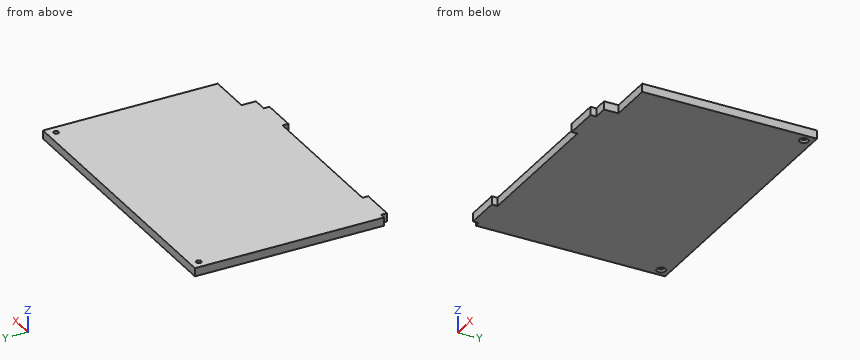
from build123d import *

# Parameters (mm, degrees)
BOSS_EXTRUDE1_DEPTH                             = 5.9
MOVE_FACE1_BY                                   = 6.3
CSK_FOR_M3_FLAT_HEAD_MACHINE_SCREW2_D           = 3.6
CSK_FOR_M3_FLAT_HEAD_MACHINE_SCREW2_CSINK_D     = 6.3
CSK_FOR_M3_FLAT_HEAD_MACHINE_SCREW2_CSINK_ANGLE = 90


with BuildPart() as part:
    # Sketch1 → Boss-Extrude1 (new body)
    with BuildSketch(Plane.XY):
        Polygon((0, 0), (10.125, 0), (10.125, -4.1), (34.625, -4.1), (34.625, 0), (138.875, 0), (138.875, -4.1), (163.375, -4.1), (163.375, 0), (173.5, 0), (173.5, 10.25), (204.5, 10.25), (204.5, 134.25), (0, 134.25), align=None)
    extrude(amount=BOSS_EXTRUDE1_DEPTH)

    # Move Face1: a face moved inward by 6.3
    extrude(part.faces().sort_by_distance((0, 67.125, 2.95))[0], amount=MOVE_FACE1_BY, dir=(1, 0, 0), mode=Mode.SUBTRACT)

    # CSK for M3 Flat Head Machine Screw2 (through all)
    with Locations(Plane(origin=(0, 0, 0), x_dir=(-1, 0, 0), z_dir=(0, 0, -1))):
        with Locations((-198.5, 128.25), (-12.3, 128.25)):
            CounterSinkHole(CSK_FOR_M3_FLAT_HEAD_MACHINE_SCREW2_D / 2, CSK_FOR_M3_FLAT_HEAD_MACHINE_SCREW2_CSINK_D / 2, counter_sink_angle=CSK_FOR_M3_FLAT_HEAD_MACHINE_SCREW2_CSINK_ANGLE)


solid = part.part
CAD build for the part. Positions are in the model's coordinates, mm. Coordinates: 2 decimals unless noted, no trailing zeros. Loops run counter-clockwise (first coordinate to the right, second up) from the corner with the lowest first, then second, coordinate; pieces in that order, holes last. Notation, with made-up numbers: (47, 74.5) -> (78, 74.5) arc R19 ccw to (78, 95.5) -> close; hole circle Ø1 at (-25.75, 80). An arc over 180 degrees is marked (long way). One line per item, written item: value.
1. Flat gauge pins, fed straight in: P1, Ø4, axis at x = 198.5, y = 128.25, coming from the -Z side; P2, Ø1.2, axis at y = -2.5, z = 3, coming from the -X side (3 decimals); P3, Ø1.8, axis at x = 74, z = 2, coming from the -Y side. Where does each tip first touch, or does it go through?
Answers:
P1: stops at z = 1.15
P2: stops at x = 10.125
P3: stops at y = 0
2. Drill centre lines: line 1 (X direction, y = 128.25, z = 4); line 2 (Y direction, x = 12.3, z = 2.45); line 3 (Y direction, x = 127.5, z = 2.2). Where is each one in solid material? Low to high. Write a range as [from, to].
Answers:
line 1: x = [6.3, 10.5], [14.1, 196.7], [200.3, 204.5]
line 2: y = [-4.1, 126.45], [130.05, 134.25]
line 3: y = [0, 134.25]
3. Slice it at B-B on x = 186. Write the cut outline in (y, z).
Answers:
outline: (10.25, 0) -> (134.25, 0) -> (134.25, 5.9) -> (10.25, 5.9) -> close
4. Slice it at C-C on x = 108.5. Write the cut outline in (y, z), and give its area (3 significant figures).
Answers:
outline: (0, 0) -> (134.25, 0) -> (134.25, 5.9) -> (0, 5.9) -> close
area: 792 mm^2
5. Slice it at A-A on z = 4.75. Write the cut outline in (x, y) (3 decimals).
Answers:
outline: (6.3, 0) -> (10.125, 0) -> (10.125, -4.1) -> (34.625, -4.1) -> (34.625, 0) -> (138.875, 0) -> (138.875, -4.1) -> (163.375, -4.1) -> (163.375, 0) -> (173.5, 0) -> (173.5, 10.25) -> (204.5, 10.25) -> (204.5, 134.25) -> (6.3, 134.25) -> close; hole circle Ø3.6 at (12.3, 128.25); hole circle Ø3.6 at (198.5, 128.25)
